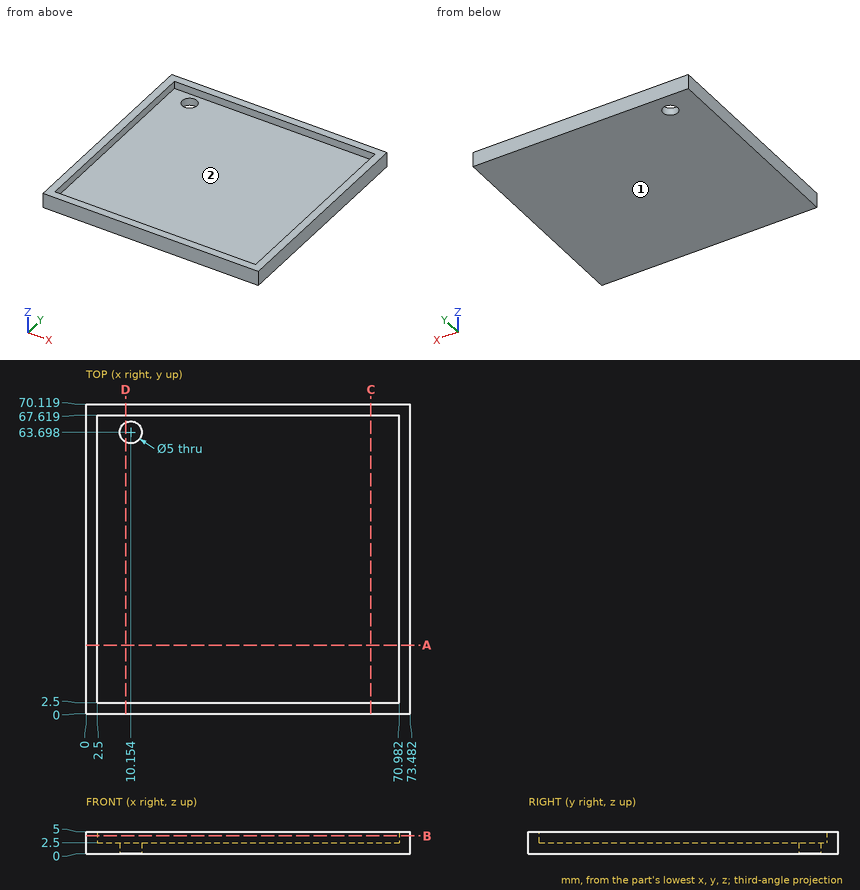
Answer from the drawing. Dimensions are ordinates in mm from the lowest x, y and z of the part. Coordinates: 2 decimals unless noted, no trailing zeros. Write each loop counter-clockwise with the first axis right and the second up, starting at its lowest first coordinate (ties: lowest second). Pieces come first, ordered by that corner, then holes. Notation, with made-up numbers: (-23.75, 26) - (6.25, 26) arc R36 ccw to (6.25, 61) - close; hole circle Ø2 at (-6.75, -27). An arc over 180 degrees is marked (long way). Return JSON: item names as keys, results as strings.
1. The part is cut by section A-A on y = 15.5. Determine the outline of the cut face in (x, z).
Final values:
{"outline": "(0, 0) - (73.48, 0) - (73.48, 5) - (70.98, 5) - (70.98, 2.5) - (2.5, 2.5) - (2.5, 5) - (0, 5) - close"}
2. This flat-tipped pin is pushed along its axis until it touches: pin 1 Ø5 at (x, y) = (44, 36.5) entering from +Z. Where does it stop, or does it pass through?
Final values:
{"pin 1": "z = 2.5"}
3. The part is cut by section C-C on x = 64.5. Determine the outline of the cut face in (y, z), then the cut area to 3 significant figures.
Final values:
{"outline": "(0, 0) - (70.12, 0) - (70.12, 5) - (67.62, 5) - (67.62, 2.5) - (2.5, 2.5) - (2.5, 5) - (0, 5) - close", "area": "188 mm^2"}
4. The part is cut by section D-D on x = 9. Determine the outline of the cut face in (y, z) (1 decimal).
Final values:
{"outline": "(0, 0) - (61.5, 0) - (61.5, 2.5) - (2.5, 2.5) - (2.5, 5) - (0, 5) - close; (65.9, 0) - (70.1, 0) - (70.1, 5) - (67.6, 5) - (67.6, 2.5) - (65.9, 2.5) - close"}
5. For a pull along X with two mould halves and no side action, classify the marked faces 1 and 2 as +X half, -X half, draft (parallel to the pull), parting line (faces both ways), or undercut.
Final values:
{"face 1": "draft", "face 2": "undercut"}
6. Consider line 1 along X through (y, z) = (11.5, 3.55); line 2 along Y through (x, z) = (12, 4); line 3 along Z through (x, y) = (69.5, 5). Determine where each line is inside the solid, lowest interval first.
Final values:
{"line 1": "0 to 2.5, 70.98 to 73.48", "line 2": "0 to 2.5, 67.62 to 70.12", "line 3": "0 to 2.5"}
7. The part is cut by section B-B on z = 4. Determine the outline of the cut face in (x, y).
Final values:
{"outline": "(0, 0) - (73.48, 0) - (73.48, 70.12) - (0, 70.12) - close; hole (2.5, 2.5) - (70.98, 2.5) - (70.98, 67.62) - (2.5, 67.62) - close"}
